Source: CAD feature listing. Evaluate the final solid. Frame: model axes, mm. Face numbers are marked on the shaded views. A direction names the side the tool comes from. Give positions to 0.01 mm unless a question says otherwise; leave off trailing zeros. Order: outer loops, then holes, each group sorted by start corner. A loop starts at its lowest first (then second) coordinate and runs counter-clockwise, first axis right, second up.
1) Material intervals for line 1 (Z direction, x = 12.7, y = 1.35); line 2 (X direction, y = 17, z = 95.5) (3 decimals), sorted ascending.
2) Section A-A, the plane x = 12.7. Return loops of the section in (y, z) (1 decimal).
3) Section D-D, the plane x = 19. Return loops of the section in (y, z) (3 decimals).
4) Section B-B, the plane y = 2.25. Return loops of the section in (x, z), plus the area to 3 significant figures.
5) Access query for the marked faces 1 and 2. Directions: +Z, -Z, +X, -X, +Y, -Y. A direction counts if a zero-diameter tool reaches every point of the face in a straight line with its end or side. Return the directions, or none.
6) Section C-C, the plane y = 15. Return loops of the section in (x, z) (3 decimals), plus the area to 3 significant figures.
7) First-contact query: P1, Ø4, axis at y = 7, z = 71, coming from the +X side; P2, Ø12, axis at y = 15.5, z = 41.5, coming from the +X side (3 decimals); P3, Ø9, axis at x = 12.7, z = 12.7, coming from the +Y side (3 decimals). Flat tips, straight axial feed; report the tip coordinate or a pass-through.
Autodesk Inventor part; units mm, degrees
ref_plane "YZ Plane" through (0, 0, 0) normal (1, 0, 0) x (0, 1, 0)
ref_plane "XZ Plane" through (0, 0, 0) normal (0, 1, 0) x (-1, 0, 0)
ref_plane "XY Plane" through (0, 0, 0) normal (0, 0, 1) x (1, 0, 0)
sketch "Sketch1" plane through (0, 0, 0) normal (0, 0, 1) x (1, 0, 0)
  line L0 (0, 25.4) -> (0, 0)
  line L1 (0, 0) -> (25.4, 0)
  line L2 (25.4, 0) -> (25.4, 3.175)
  line L3 (25.4, 3.175) -> (3.175, 3.175)
  line L4 (3.175, 3.175) -> (3.175, 25.4)
  line L5 (3.175, 25.4) -> (0, 25.4)
  dimension "d0" = 25.4
  dimension "d1" = 25.4
  dimension "d2" = 3.175
  dimension "d3" = 3.175
extrude "Extrusion1" add sketch "Sketch1" along normal blind 101.6
fillet "Fillet1" radius 3.175 1 edges at (3.175, 3.175, 50.8)
hole "Hole1" at (12.7, 3.175, 88.9) direction (0, -1, 0) diameter 6.731 end through all
pattern_linear "Rectangular Pattern1" count 2 spacing 76.2 along (0, 0, -1) of "Hole1"
fillet "Fillet3" radius 2.3876 2 edges at (3.175, 25.4, 50.8) (25.4, 3.175, 50.8)
sketch "Sketch2" plane through (3.175, 6.35, 101.6) normal (1, 0, 0) x (0, 0, -1)
  line L0 (0, 16.6624) -> (0, 0)
  line L1 (101.6, 16.6624) -> (101.6, 0)
  arc A0 (25.4, 12.8905) -> (25.4, 6.1595) centre (25.4, 9.525) ccw
  arc A1 (31.75, 6.1595) -> (31.75, 12.8905) centre (31.75, 9.525) ccw
  arc A2 (69.85, 12.8905) -> (69.85, 6.1595) centre (69.85, 9.525) ccw
  arc A3 (76.2, 6.1595) -> (76.2, 12.8905) centre (76.2, 9.525) ccw
  line L2 (25.4, 12.8905) -> (31.75, 12.8905)
  line L3 (31.75, 6.1595) -> (25.4, 6.1595)
  line L4 (69.85, 12.8905) -> (76.2, 12.8905)
  line L5 (76.2, 6.1595) -> (69.85, 6.1595)
  line L6 (101.6, -6.35) -> (0, -6.35)
  dimension "d21" = 6.731
  dimension "d22" = 6.35
  dimension "d23" = 6.35
  dimension "d24" = 15.875
  dimension "d25" = 15.875
  dimension "d26" = 25.4
  dimension "d27" = 25.4
extrude "Extrusion2" cut sketch "Sketch2" against normal blind 25.4
properties part number "GE-12102"
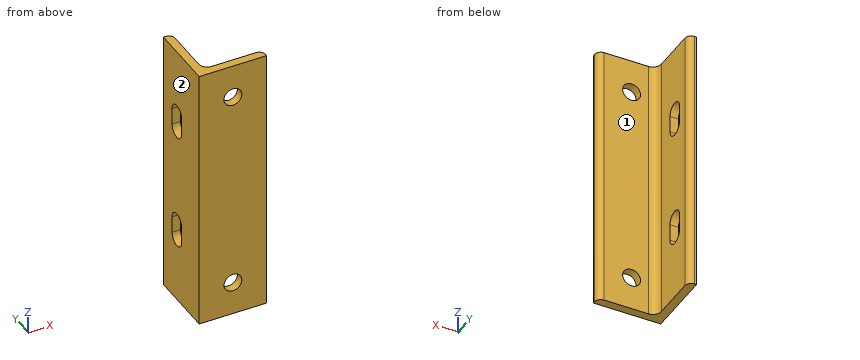
From the geometry:
1. line 1: z = 0 to 9.33, 16.07 to 85.53, 92.27 to 101.6
1. line 2: x = 0 to 3.175
2. outline: (0, 0) - (3.2, 0) - (3.2, 9.3) - (0, 9.3) - close; (0, 16.1) - (3.2, 16.1) - (3.2, 85.5) - (0, 85.5) - close; (0, 92.3) - (3.2, 92.3) - (3.2, 101.6) - (0, 101.6) - close
3. outline: (0, 0) - (3.175, 0) - (3.175, 101.6) - (0, 101.6) - close
4. outline: (0, 0) - (24.9, 0) - (24.9, 101.6) - (0, 101.6) - close; hole circle Ø6.73 at (12.7, 12.7); hole circle Ø6.73 at (12.7, 88.9)
4. area: 2,460 mm2
5. face 1: +Z, -Z, +X, +Y
5. face 2: +Z, -Z, -X, +Y, -Y
6. outline: (0, 0) - (3.175, 0) - (3.175, 22.15) - (0, 22.15) - close; (0, 35) - (3.175, 35) - (3.175, 66.6) - (0, 66.6) - close; (0, 79.45) - (3.175, 79.45) - (3.175, 101.6) - (0, 101.6) - close
6. area: 241 mm2
7. P1: stops at x = 3.48
7. P2: stops at x = 3.175
7. P3: stops at y = 3.175
